Build history of the part. All positions in model axes, mm. A direction names the side the tool comes from. Round coordinates to 2 decimals unless told otherwise and drop trailing zeros. Write each loop counter-clockwise with the first axis right and the second up, starting at its lowest first coordinate (ties: lowest second). Pieces come first, ordered by that corner, then holes. Notation, with made-up numbers: (58.5, 57.5) - (104.5, 57.5) arc R22 ccw to (104.5, 78.5) - close; hole circle Ø2 at (-20, 24.25). An arc over 180 degrees is marked (long way). Answer as a JSON object with one key per item and string values. Group by question number.
Item 1: Probe line 1 (Z direction, x = 41, y = 9.75) (3 decimals); line 2 (X direction, y = 5, z = 0.75); line 3 (X direction, y = 7, z = -0.5). List the from-to ranges inside material, lowest first. Write a range as from..to.
Item 2: Flat gauge pins, fed straight in: pin 1 (3 mm diameter, centred on x = 0, z = 0, fed in from -Y); pin 2 (3 mm diameter, centred on x = 30.5, z = 0, fed in from +Y); pin 3 (1.5 mm diameter, centred on y = 5.5, z = -0.5, fed in from +X). Where does each tip first touch, or does it go through?
Item 3: Slice it at D-D, the plane y = 3.75. List the corners of the cut face in (x, z) (1 decimal).
Item 4: Slice it at C-C, the plane x = 0. List the corners of the cut face in (y, z) (1 decimal), then the cut area to 3 significant figures.
Item 5: Two-plate mould, pull along Z, no slides. Class faces 1 (the flat face through (43.688, 3, 0)), 2 (the flat face through (41, 11.43, 0)), 3 (the flat face through (-1, 13, 3.175)): +Z half, -Z half, draft (parallel to the pull), parting line (faces both ways), or undercut.
Item 6: Slice it at A-A, the plane y = 7.25. List the corners of the cut face in (x, z) (1 decimal), then the cut area to 3 significant figures.
Item 7: Which spindle directions (+Z, -Z, +X, -X, +Y, -Y) get a long thin tool onto all of the face, cutting with end or side? Do faces 4 (the flat face through (44.323, 10, 0)), 5 (the flat face through (25, 14.288, 0)), 6 (the cylindrical face through (42.099, 5.635, -1.047)), 7 (the flat face through (-43.688, 3, 0)). Say none if no direction does.
Autodesk Inventor part; units mm, degrees
ref_plane "YZ Plane" through (0, 0, 0) normal (1, 0, 0) x (0, 1, 0)
ref_plane "XZ Plane" through (0, 0, 0) normal (0, 1, 0) x (-1, 0, 0)
ref_plane "XY Plane" through (0, 0, 0) normal (0, 0, 1) x (1, 0, 0)
sketch "Sketch1" plane through (0, 0, 0) normal (0, 0, 1) x (1, 0, 0)
  line L0 (-44.323, 14.2875) -> (44.323, 14.2875)
  line L1 (44.323, 14.2875) -> (44.323, -14.2875)
  line L2 (44.323, -14.2875) -> (-44.323, -14.2875)
  line L3 (-44.323, -14.2875) -> (-44.323, 14.2875)
  point P0 (0, 0)
  dimension "d0" = 88.646
  dimension "d1" = 44.323
  dimension "d2" = 14.2875
  dimension "d3" = 28.575
extrude "Extrusion1" add sketch "Sketch1" along normal mid plane 6.35
sketch "Sketch2" plane through (0, 0, 3.175) normal (0, 0, 1) x (1, 0, 0)
  circle A0 centre (-26.924, 0) radius 11.303
  circle A1 centre (0, 0) radius 11.303
  line L0 (44.323, -14.2875) -> (44.323, 14.2875)
  circle A2 centre (26.924, 0) radius 11.303
  line L1 (-44.323, 14.2875) -> (-44.323, -14.2875)
  line L2 (-44.323, 0) -> (44.323, 0) construction
  line L3 (44.323, 14.2875) -> (-44.323, 14.2875)
  point P0 (0, 0)
  dimension "d6" = 22.606
  dimension "d9" = 22.606
  dimension "d11" = 22.606
  dimension "d14" = 26.924
  dimension "d21" = 88.646
  dimension "d22" = 26.924
  dimension "d45" = 0
sketch "Sketch4" plane through (-44.323, -14.2875, -3.175) normal (-1, 0, 0) x (0, 0, 1)
  line L0 (0, 0) -> (0, 28.575)
  line L1 (6.35, 28.575) -> (6.35, 0)
  line L2 (0, 22.6695) -> (6.35, 22.6695)
  line L3 (6.35, 22.6695) -> (6.35, 5.9055)
  line L4 (6.35, 5.9055) -> (0, 5.9055)
  line L5 (0, 5.9055) -> (0, 22.6695)
  point P0 (3.175, 14.2875)
  dimension "d30" = 8.382
  dimension "d31" = 16.764
extrude "Extrusion3" cut sketch "Sketch4" against normal blind 0.635
mirror "Mirror1" about plane through (0, 0, 0) normal (1, 0, 0) of "Extrusion3"
sketch "Sketch7" plane through (-44.323, -14.2875, 3.175) normal (0, -1, 0) x (1, 0, 0)
  line L0 (30.353, -14.605) -> (58.293, -14.605)
  line L1 (58.293, -14.605) -> (58.293, 8.255)
  line L2 (58.293, 8.255) -> (30.353, 8.255)
  line L3 (30.353, 8.255) -> (30.353, -14.605)
  point P0 (44.323, -3.175)
  dimension "d39" = 27.94
  dimension "d40" = 22.86
  dimension "d41" = 11.43
  dimension "d42" = 13.97
extrude "Extrusion5" [suppressed]
extrude "Extrusion6" cut sketch "Sketch2" against normal blind 25.4
sketch "Sketch8" plane through (0, 0, -3.175) normal (0, 0, -1) x (-1, 0, 0)
  line L0 (43.688, 8.382) -> (43.688, -8.382) construction
  line L1 (43.688, 0) -> (-43.688, 0)
  line L2 (-43.688, 8.382) -> (-43.688, -8.382) construction
  line L3 (44.323, 14.2875) -> (-44.323, 14.2875)
  line L4 (44.323, 8.382) -> (44.323, 14.2875)
  line L5 (-44.323, 14.2875) -> (-44.323, 8.382)
  line L6 (-43.688, 8.382) -> (-43.688, 0)
  line L7 (-44.323, 8.382) -> (-43.688, 8.382)
  line L8 (43.688, 8.382) -> (43.688, 0)
  line L9 (43.688, 8.382) -> (44.323, 8.382)
  point P0 (0, 0)
extrude "Extrusion7" [suppressed]
sketch "Sketch9" plane through (0, 0, -3.175) normal (0, 0, -1) x (-1, 0, 0)
  line L0 (-44.323, -14.2875) -> (44.323, -14.2875)
  line L1 (44.323, -14.2875) -> (44.323, -8.382)
  line L2 (44.323, -8.382) -> (43.688, -8.382)
  line L3 (-43.688, -8.382) -> (-44.323, -8.382)
  line L4 (-44.323, -8.382) -> (-44.323, -14.2875)
  line L5 (-43.688, 8.382) -> (-43.688, -8.382)
  line L6 (-43.688, 0) -> (-43.688, -8.382)
  line L7 (-43.688, 0) -> (43.688, 0)
  line L8 (43.688, -8.382) -> (43.688, 8.382)
  line L9 (43.688, -8.382) -> (43.688, 0)
  point P0 (0, 0)
extrude "Extrusion8" cut sketch "Sketch9" against normal through all
sketch "Sketch10" plane through (-43.688, 0, -3.175) normal (0, -1, 0) x (1, 0, 0)
  line L0 (5.461, 6.35) -> (5.461, 0)
  line L1 (0, 0) -> (0, 6.35)
  line L2 (-0.635, 0) -> (-0.635, 6.35)
  line L3 (5.461, 6.35) -> (5.461, 0)
  line L4 (0, 6.35) -> (5.461, 6.35)
  line L5 (0, 0) -> (0, 6.35)
  line L6 (5.461, 0) -> (0, 0)
  circle A0 centre (2.7305, 3.175) radius 1.5494
  line L7 (86.614, 1.27) -> (80.264, 1.27)
  line L8 (86.614, 0) -> (80.264, 0)
  point P0 (43.688, 3.175)
  point P1 (84.328, 1.27)
  point P2 (77.978, 1.27)
  point P3 (84.328, 0)
  point P4 (77.978, 0)
  dimension "d58" = 3.0988
  dimension "d61" = 5.461
  dimension "d62" = 2.7305
  dimension "d78" = 3.175
  dimension "d90" = 6.35
extrude "Extrusion9" cut sketch "Sketch10" against normal blind 11.43 contours A0
mirror "Mirror2" about plane through (0, 0, 0) normal (1, 0, 0) of "Extrusion9"
thread "Thread1"
thread "Thread2"
fillet "Fillet1" radius 3.175 2 edges at (-44.323, 14.2875, 0) (44.323, 14.2875, 0)
sketch "Sketch12" plane through (-41.148, 14.2875, -3.175) normal (0, 1, 0) x (1, 0, 0)
  line L0 (82.296, -6.35) -> (0, -6.35)
  line L1 (34.798, 0) -> (47.498, 0)
  line L2 (47.498, 0) -> (47.498, -6.35)
  line L3 (47.498, -6.35) -> (34.798, -6.35)
  line L4 (34.798, -6.35) -> (34.798, 0)
  circle A0 centre (41.148, -3.175) radius 1
  line L5 (29.845, 0) -> (52.451, 0)
  dimension "d81" = 6.35
  dimension "d82" = 12.7
  dimension "d83" = 2
  dimension "d87" = 0
extrude "Extrusion11" add sketch "Sketch12" along normal blind 3.8
fillet "Fillet3" radius 3.175 2 edges at (6.35, 14.2875, 0) (-6.35, 14.2875, 0)
thread "Thread3"
fillet "Fillet4" radius 3.175 2 edges at (43.688, 8.382, 0) (-43.688, 8.382, 0)
equation "\"d9\" = d7"
equation "\"d11\" = d9"
equation "\"d22\" = d14"
equation "\"d62\" = 0.5 * d61"
equation "\"d78\" = 0.5 * d90"
equation "\"d7\" = d6"
properties part number "Tube Holder Halve 2" material "Aluminum 6061-AHC"
Geometry says:
{
 "1": {"line 1": "z = -3.175..-1.549, 1.549..3.175", "line 2": "x = -43.69..-42.31, -39.6..-37.06, -16.79..-10.14, 10.14..16.79, 37.06..39.6, 42.31..43.69", "line 3": "x = -43.73..-42.42, -39.49..-35.8, -18.05..-8.87, 8.87..18.05, 35.8..39.49, 42.42..43.73"},
 "2": {"pin 1": "stops at y = 11.2", "pin 2": "stops at y = 14.29", "pin 3": "stops at x = 43.69"},
 "3": {"outline": "(-43.7, -3.2) - (-37.6, -3.2) - (-37.6, 3.2) - (-43.7, 3.2) - close; (-16.3, -3.2) - (-10.7, -3.2) - (-10.7, 3.2) - (-16.3, 3.2) - close; (10.7, -3.2) - (16.3, -3.2) - (16.3, 3.2) - (10.7, 3.2) - close; (37.6, -3.2) - (43.7, -3.2) - (43.7, 3.2) - (37.6, 3.2) - close; hole circle Ø3.1 at (-41, 0); hole circle Ø3.1 at (41, 0)"},
 "4": {"outline": "(11.3, -3.2) - (18.1, -3.2) - (18.1, -1) - (14.3, -1) - (14.3, 1) - (18.1, 1) - (18.1, 3.2) - (11.3, 3.2) - close", "area": "35.5 mm^2"},
 "5": {"face 1": "draft", "face 2": "undercut", "face 3": "+Z half"},
 "6": {"outline": "(-43.8, -3.2) - (-35.6, -3.2) - (-35.6, 3.2) - (-43.8, 3.2) - close; (-18.3, -3.2) - (-8.7, -3.2) - (-8.7, 3.2) - (-18.3, 3.2) - close; (8.7, -3.2) - (18.3, -3.2) - (18.3, 3.2) - (8.7, 3.2) - close; (35.6, -3.2) - (43.8, -3.2) - (43.8, 3.2) - (35.6, 3.2) - close; hole circle Ø3.1 at (-41, 0); hole circle Ø3.1 at (41, 0)", "area": "211 mm^2"},
 "7": {"face 4": "+Z, -Z, +X, +Y, -Y", "face 5": "+Z, -Z, +X, +Y", "face 6": "-Y", "face 7": "+Z, -Z, -X, -Y"}
}
